```python
from build123d import *

# Parameters (mm, degrees)
SKETCH1_W           = 15
SKETCH1_H           = 15
BOSS_EXTRUDE1_DEPTH = 4
SKETCH3_R           = 4.037394367
CUT_EXTRUDE2_DEPTH  = 1
SKETCH2_R           = 4.037394367
CUT_EXTRUDE3_DEPTH  = 2


with BuildPart() as part:
    # Sketch1 → Boss-Extrude1 (new body)
    with BuildSketch(Plane(origin=(0, 0, 0), x_dir=(1, 0, 0), z_dir=(0, 1, 0))):
        with Locations((-3.092315207, 3.037793064)):
            Rectangle(SKETCH1_W, SKETCH1_H)
    extrude(amount=BOSS_EXTRUDE1_DEPTH)

    # Sketch3 → Cut-Extrude2 (cut)
    with BuildSketch(Plane(origin=(0, 4, 0), x_dir=(1, 0, 0), z_dir=(0, 1, 0))):
        Circle(SKETCH3_R)
        with BuildLine():
            Line((-2.029498636, -0.179195686), (-1.109423018, -0.097957109))
            Line((-1.109423018, -0.097957109), (1.710275386, 1.107218999))
            ThreePointArc((1.710275386, 1.107218999), (-0.662715291, 1.926599141), (-2.029498636, -0.179195686))
        make_face(mode=Mode.SUBTRACT)
        with BuildLine():
            Line((1.987822429, 0.44669654), (-0.18326754, -0.467866029))
            Line((-0.18326754, -0.467866029), (-1.709632143, -1.108211957))
            ThreePointArc((-1.709632143, -1.108211957), (0.789799068, -1.87808233), (1.987822429, 0.44669654))
        make_face(mode=Mode.SUBTRACT)
    extrude(amount=-CUT_EXTRUDE2_DEPTH, mode=Mode.SUBTRACT)

    # Sketch2 → Cut-Extrude3 (cut)
    with BuildSketch(Plane(origin=(0, 4, 0), x_dir=(1, 0, 0), z_dir=(0, 1, 0))):
        with Locations((-6.070431837, 6.178975723)):
            Circle(SKETCH2_R)
        with BuildLine():
            Line((-8.099930473, 5.999780036), (-7.179854855, 6.081018614))
            Line((-7.179854855, 6.081018614), (-4.360156451, 7.286194722))
            ThreePointArc((-4.360156451, 7.286194722), (-6.733147128, 8.105574864), (-8.099930473, 5.999780036))
        make_face(mode=Mode.SUBTRACT)
        with BuildLine():
            Line((-4.082609408, 6.625672263), (-6.253699377, 5.711109693))
            Line((-6.253699377, 5.711109693), (-7.78006398, 5.070763766))
            ThreePointArc((-7.78006398, 5.070763766), (-5.280632769, 4.300893392), (-4.082609408, 6.625672263))
        make_face(mode=Mode.SUBTRACT)
    extrude(amount=-CUT_EXTRUDE3_DEPTH, mode=Mode.SUBTRACT)


solid = part.part
```
Can you work these out from the model? Positions are in its coordinate system, mm. A direction names the side the tool comes from. Coordinates: 2 decimals unless noted, no trailing zeros. Order: outer loops, then holes, each group sorted by start corner. A loop starts at its lowest first (then second) coordinate and runs counter-clockwise, first axis right, second up. Notation, with made-up numbers: (45.25, 4.5) -> (66.25, 4.5) arc R21 ccw to (66.25, 32.5) -> close; hole circle Ø10 at (81, -7). An arc over 180 degrees is marked (long way). Write each question's results on one line, items separated by ' | '.
Item 1: I want a section at C-C, the plane x = 0.25. Write out the boundary of the cut face in (y, z).
Results are:
outline: (0, -10.54) -> (4, -10.54) -> (4, -4.03) -> (3, -4.03) -> (3, -2.02) -> (4, -2.02) -> (4, -0.48) -> (3, -0.48) -> (3, 0.29) -> (4, 0.29) -> (4, 2.02) -> (3, 2.02) -> (3, 4.03) -> (4, 4.03) -> (4, 4.46) -> (0, 4.46) -> close
Item 2: I want a section at A-A, the plane y = 2.8. Write out the boundary of the cut face in (x, z), then the cut area to 3 significant figures.
Results are:
outline: (-10.59, -10.54) -> (4.41, -10.54) -> (4.41, 4.46) -> (-10.59, 4.46) -> close; (-8.1, -6) arc R2.04 ccw to (-4.36, -7.29) -> (-7.18, -6.08) -> close; (-7.78, -5.07) -> (-6.25, -5.71) -> (-4.08, -6.63) arc R2.04 ccw to start; hole circle Ø8.07 at (-6.07, -6.18) | area: 184 mm²
Item 3: I want a section at D-D, the plane x = 3.25. Write out the boundary of the cut face in (y, z), then the cut area to 3 significant figures.
Results are:
outline: (0, -10.54) -> (4, -10.54) -> (4, -2.4) -> (3, -2.4) -> (3, 2.4) -> (4, 2.4) -> (4, 4.46) -> (0, 4.46) -> close | area: 55.2 mm²
Item 4: Which directions (+Z, -Z, +X, -X, +Y, -Y) give clear straight access to the entire face, cutting with the end or side of a thin tool? Please do faces 1 (the face through (-3, 2, -10.538)), 2 (the face through (-6, 2, -6)).
Results are:
face 1: -Z, +X, -X, +Y, -Y | face 2: +Y
Item 5: If I drill on line 1 along X through (y, z) = (3.5, 1.25); line 2 along X through (y, z) = (3.55, -5.75); line 3 along Z through (x, y) = (1.25, 3.15), over which ranges is the centre line in solid material (lowest first)?
Results are:
line 1: -10.59 to -3.84, -1.61 to 1.61, 3.84 to 4.41 | line 2: -10.59 to -10.08, -6.16 to -4.08, -2.06 to 4.41 | line 3: -10.54 to -3.84, -1.61 to -0.91, -0.14 to 1.61, 3.84 to 4.46
Item 6: I want a section at B-B, the plane x = -3.5. Write out the boundary of the cut face in (y, z).
Results are:
outline: (0, -10.54) -> (4, -10.54) -> (4, -9.29) -> (2, -9.29) -> (2, -3.07) -> (4, -3.07) -> (4, -2.01) -> (3, -2.01) -> (3, 2.01) -> (4, 2.01) -> (4, 4.46) -> (0, 4.46) -> close
Item 7: If we mould it in two halves opening along X, with no side actions, what happens to faces 3 (the face through (4.408, 2, -3)), 4 (the face through (0.753, 3.507, 1.893)), 5 (the face through (-3, 4, -3)), 6 (the face through (0.917, 3.507, 0.004))? For each: +X half, -X half, draft (parallel to the pull), parting line (faces both ways), or undercut.
Results are:
face 3: +X half | face 4: undercut | face 5: draft | face 6: undercut
